from build123d import *

# Parameters (mm, degrees)
SKETCH1_R           = 26.5
BOSS_EXTRUDE1_DEPTH = 10.5
BOSS_EXTRUDE2_START = -2.5
SKETCH1_3_R         = 28
SKETCH1_3_R_2       = 27.5
SKETCH1_3_R_3       = 26.5
BOSS_EXTRUDE2_DEPTH = 2.5
BOSS_EXTRUDE3_START = -6.5
SKETCH1_4_R         = 27.5
SKETCH1_4_R_2       = 26.5
BOSS_EXTRUDE3_DEPTH = 6.5


with BuildPart() as part:
    # Sketch1 → Boss-Extrude1 (new body)
    with BuildSketch(Plane(origin=(0, 0, 0), x_dir=(1, 0, 0), z_dir=(0, 1, 0))):
        with Locations(Location((0, 0, 0), (0, 0, 90))):
            Circle(SKETCH1_R)
    extrude(amount=BOSS_EXTRUDE1_DEPTH)

    # Sketch1_3 → Boss-Extrude2 (add)
    # profile 1 of 3: a face of its own
    with BuildSketch(Plane(origin=(0, 0, 0), x_dir=(1, 0, 0), z_dir=(0, 1, 0)).offset(BOSS_EXTRUDE2_START)):
        with Locations(Location((0, 0, 0), (0, 0, 270))):
            Circle(SKETCH1_3_R)
        Circle(SKETCH1_3_R_2, mode=Mode.SUBTRACT)
    # profile 2 of 3: a face of its own
    with BuildSketch(Plane(origin=(0, 0, 0), x_dir=(1, 0, 0), z_dir=(0, 1, 0)).offset(BOSS_EXTRUDE2_START)):
        Circle(SKETCH1_3_R_2)
        with Locations(Location((0, 0, 0), (0, 0, 90))):
            Circle(SKETCH1_3_R_3, mode=Mode.SUBTRACT)
    # profile 3 of 3: a face of its own
    with BuildSketch(Plane(origin=(0, 0, 0), x_dir=(1, 0, 0), z_dir=(0, 1, 0)).offset(BOSS_EXTRUDE2_START)):
        with Locations(Location((0, 0, 0), (0, 0, 90))):
            Circle(SKETCH1_3_R_3)
    extrude(amount=BOSS_EXTRUDE2_DEPTH)

    # Sketch1_4 → Boss-Extrude3 (add)
    with BuildSketch(Plane(origin=(0, 0, 0), x_dir=(1, 0, 0), z_dir=(0, 1, 0)).offset(BOSS_EXTRUDE3_START)):
        with Locations(Location((0, 0, 0), (0, 0, 270))):
            Circle(SKETCH1_4_R)
        with Locations(Location((0, 0, 0), (0, 0, 90))):
            Circle(SKETCH1_4_R_2, mode=Mode.SUBTRACT)
    extrude(amount=BOSS_EXTRUDE3_DEPTH)


solid = part.part
The model under review builds one solid part; all positions refer to its coordinate system, in mm. A direction names the side the tool comes from. Give positions to 0.01 mm unless a question says otherwise; leave off trailing zeros. Order: outer loops, then holes, each group sorted by start corner. A loop starts at its lowest first (then second) coordinate and runs counter-clockwise, first axis right, second up. Notation, with made-up numbers: M 63,-33 L 84,-33 A19 cw 84,-10 Z; hole C -10.5,41.5 d1. An arc over 180 degrees is marked long. One line per question, with ' | ' between items. Start each with the question number.
1) Consider section B-B, the plane x = 0. Give the boundary of the cut face in (y, z).
2) Wall thickness on L1, parallel to X at y = -5.55, z = 0; L2, parallel to Y at x = 7, z = -16; L3, parallel to Z at x = -13, y = -2.75: over which ranges is each line inside the solid? List them lowest first. Write a range as from..to.
3) Consider section A-A, the plane z = 0. Give the boundary of the cut face in (x, y).
4) Mouldability with a two-part tool opening along Z and no side actions: class faces 1 (the face through (14, -6.5, -23)), 2 (the face through (-26.274, -4.528, 3.45)), 3 (the face through (-27.334, -1.268, -6.07)) as pulls with the +Z half, pulls with the -Z half, needs draft (parallel to the pull), parting line crosses it, or undercut.
5) For faces 4 (the face through (-26.274, 5.176, 3.45)), 5 (the face through (-24.397, -4.528, 12.69)), 6 (the face through (0, 10.5, 0)), list the 3-axis set-ups (+Z, -Z, +X, -X, +Y, -Y) from which the entire face can be reached by the end or side of a thin tool; tool diameter is ignored.
6) Consider section C-C, the plane y = 1.75. Give the boundary of the cut face in (x, z).
7) Clearance check with flat-ended pins moving along their axes: P1, Ø5, axis at x = -8.5, y = -3.5, coming from the -Z side; P2, Ø6, axis at x = -21, y = 7.5, coming from the +Z side; P3, Ø3, axis at y = 8.5, z = 6.5, coming from the +X side. State where each tip first meets the part, or that it passes through.
8) Consider section D-D, the plane y = -4.25. Give the boundary of the cut face in (x, z).
Found:
1) outline: M -6.5,-27.5 L -2.5,-27.5 L -2.5,-28 L 0,-28 L 0,-26.5 L 10.5,-26.5 L 10.5,26.5 L 0,26.5 L 0,28 L -2.5,28 L -2.5,27.5 L -6.5,27.5 L -6.5,26.5 L -2.5,26.5 L -2.5,-26.5 L -6.5,-26.5 Z
2) L1: x = -27.5..-26.5, 26.5..27.5 | L2: y = -2.5..10.5 | L3: z = -24.23..-23.09, 23.09..24.23
3) outline: M -28,-2.5 L -27.5,-2.5 L -27.5,-6.5 L -26.5,-6.5 L -26.5,-2.5 L 26.5,-2.5 L 26.5,-6.5 L 27.5,-6.5 L 27.5,-2.5 L 28,-2.5 L 28,0 L 26.5,0 L 26.5,10.5 L -26.5,10.5 L -26.5,0 L -28,0 Z
4) face 1: needs draft | face 2: undercut | face 3: parting line crosses it
5) face 4: +Y | face 5: -Y | face 6: +Z, -Z, +X, -X, +Y
6) outline: C 0,0 d53
7) P1: stops at z = -27.3 | P2: stops at z = 19.45 | P3: stops at x = 26.02
8) outline: C 0,0 d55; hole C 0,0 d53
